Autodesk Inventor part; units mm, degrees
ref_plane "YZ Plane" through (0, 0, 0) normal (1, 0, 0) x (0, 1, 0)
ref_plane "XZ Plane" through (0, 0, 0) normal (0, 1, 0) x (-1, 0, 0)
ref_plane "XY Plane" through (0, 0, 0) normal (0, 0, 1) x (1, 0, 0)
sketch "Esboço1" plane through (0, 0, 0) normal (0, 0, 1) x (1, 0, 0)
  line L0 (555, 651.5) -> (-555, 651.5)
  line L1 (-555, 651.5) -> (-555, -651.5)
  line L2 (-555, -651.5) -> (555, -651.5)
  line L3 (555, -651.5) -> (555, 651.5)
  point P0 (0, 0)
  point P1 (555, 0)
  point P2 (0, 651.5)
  dimension "d11" = 1110
  dimension "d12" = 1303
extrude "Extrusão1" add sketch "Esboço1" against normal blind 1700
sketch "Esboço3" plane through (-555, -651.5, 0) normal (0, -1, 0) x (1, 0, 0)
  line L0 (960, -1400) -> (250, -1400)
  line L1 (250, -1400) -> (250, -840)
  line L2 (250, -840) -> (960, -840)
  line L3 (960, -840) -> (960, -1400)
  line L4 (1110, 0) -> (1110, -1700) construction
  line L5 (0, 0) -> (0, -1700) construction
  line L6 (1110, -1700) -> (0, -1700)
  line L7 (1110, 0) -> (0, 0) construction
  point P0 (555, 0)
  dimension "d2" = 150
  dimension "d3" = 250
  dimension "d4" = 300
  dimension "d10" = 560
  dimension "d17" = 840
extrude "Extrusão2" cut sketch "Esboço3" against normal through all
chamfer "Chanfro2" distance 300 angle 45 1 edges at (555, 0, -1700)
chamfer "Chanfro1" distance 200 angle 45 2 edges at (-305, 0, -1400) (405, 0, -1400)
sketch "Esboço4" plane through (555, -651.5, 0) normal (1, 0, 0) x (0, 0, -1)
  line L0 (0, 1303) -> (0, 0)
  line L1 (660, 952.5) -> (0, 952.5)
  line L2 (0, 952.5) -> (0, 350.5)
  line L3 (0, 350.5) -> (660, 350.5)
  line L4 (660, 350.5) -> (660, 952.5)
  line L5 (0, 1303) -> (1400, 1303)
  line L6 (0, 0) -> (1400, 0)
  point P0 (0, 651.5)
  point P1 (0, 952.5)
  dimension "d19" = 350.5
  dimension "d20" = 350.5
  dimension "d21" = 660
  dimension "d22" = 602
extrude "Extrusão3" cut sketch "Esboço4" against normal blind 300
sketch "Esboço6" plane through (-555, -651.5, 0) normal (-1, 0, 0) x (0, 0, 1)
  line L0 (-660, 349) -> (0, 349)
  line L1 (0, 349) -> (0, 954)
  line L2 (0, 954) -> (-660, 954)
  line L3 (-660, 954) -> (-660, 349)
  line L4 (0, 1303) -> (0, 0)
  line L5 (0, 952.5) -> (-660, 952.5)
  point P0 (0, 651.5)
  point P1 (0, 651.5)
  dimension "d30" = 660
  dimension "d31" = 660
  dimension "d32" = 605
extrude "Extrusão5" cut sketch "Esboço6" against normal blind 300 contours L3 L5 L1 L0
shell "Casca1" thickness 1.5 removed faces 7 at (85, 534.6667, 0) at (168.3333, -217.1667, -840) at (-305, 217.1667, -960) at (-238.3333, -217.1667, -1266.6667) at (-1.6667, -217.1667, -1400) at (405, -217.1667, -1080) at (271.6667, -217.1667, -1333.3333)
sketch "Esboço5" plane through (0, 0, -1700) normal (0, 0, -1) x (-1, 0, 0)
  line L0 (55, 501.5) -> (-555, 501.5)
  line L1 (-555, 501.5) -> (-555, -501.5)
  line L2 (-555, -501.5) -> (55, -501.5)
  line L3 (55, -501.5) -> (55, 501.5)
  line L4 (-255, 651.5) -> (-555, 651.5) construction
  line L5 (-255, -651.5) -> (555, -651.5) construction
  line L6 (-555, 651.5) -> (-555, -651.5) construction
  line L7 (555, -651.5) -> (555, 651.5) construction
  line L8 (555, 651.5) -> (-555, 651.5)
  line L9 (-555, 651.5) -> (-555, -651.5)
  line L10 (-555, -651.5) -> (555, -651.5)
  line L11 (555, -651.5) -> (555, 651.5)
  point P0 (0, 0)
  dimension "d25" = 150
  dimension "d26" = 150
  dimension "d27" = 500
extrude "Extrusão4" cut sketch "Esboço5" against normal blind 800 contours L3 L2 L1 L0
sketch "Esboço7" plane through (255, -651.5, 0) normal (1, 0, 0) x (0, 0, -1)
  line L0 (661.5, 349) -> (0, 349) construction
  line L1 (440, 952.5) -> (435, 952.5)
  line L2 (435, 952.5) -> (435, 349)
  line L3 (435, 349) -> (440, 349)
  line L4 (440, 349) -> (440, 952.5)
  line L5 (0, 952.5) -> (660, 952.5) construction
  line L6 (0, 350.5) -> (0, 952.5) construction
  line L7 (660, 350.5) -> (0, 350.5) construction
  line L8 (660, 952.5) -> (660, 350.5) construction
  line L9 (0, 952.5) -> (660, 952.5)
  line L10 (215, 952.5) -> (210, 952.5)
  line L11 (210, 952.5) -> (210, 350.5)
  line L12 (210, 350.5) -> (215, 350.5)
  line L13 (215, 350.5) -> (215, 952.5)
  point P0 (0, 651.5)
  point P1 (437.5, 952.5)
  dimension "d35" = 5
  dimension "d36" = 220
  dimension "d37" = 220
equation "\"d20\" = d19"
equation "\"d26\" = d25"
equation "\"d36\" = d37"
properties part number "Croqui Célula"
For this review, take the finished solid that the model builds, in its own axes (mm). A direction names the side the tool comes from. Coordinates: 2 decimals unless noted, no trailing zeros. Write each loop counter-clockwise with the first axis right and the second up, starting at its lowest first coordinate (ties: lowest second). Pieces come first, ordered by that corner, then holes.
(1) For pin 1 Ø5 at (y, z) = (48.5, -1328) entering from +X; pin 2 Ø1 at (x, y) = (309, -138.5) entering from +Z; pin 3 Ø1.6 at (y, z) = (-108, -1699) entering from +X, all flat-tipped, find the tip position at first contact; note any pin that passes through.
(2) Add section A-A on y = -157. Give the boundary of the cut face in (x, z), then the cut area to 3 significant figures.
(3) The part is to be moulded in two halves that separate along X. For faces 1 (the face through (401.85, 574.71, -1551.03)), 2 (the face through (-246, 9, -1700)), 3 (the face through (555, -9, -690)), say which applies: +X half, -X half, draft (parallel to the pull), parting line (faces both ways), or undercut.
(4) Add section B-B on z = -1108. Give the boundary of the cut face in (x, y), then the cut area to 3 significant figures.
(5) Add section D-D on z = -326.5. Give the boundary of the cut face in (x, y).
(6) Wall thickness on probe 1 along Y at (x, z) = (-487, -189.5); probe 2 along X at (y, z) = (207, -654); probe 3 along Y at (x, z) = (-104, -93): over which ranges is each line inside the solid? List them lowest first.
(7) Tool access review of faces 4 (the face through (8, 650, -837)), 5 (the face through (406, -302.5, -326)), 6 (the face through (-407, 3, -660)): name each direction out of +Z, -Z, +X, -X, +Y, -Y from which nothing blocks a thin tool from reaching the whole face with its end or side.
(8) Add section C-C on x = -152.5. Give the boundary of the cut face in (y, z).
Answer sheet:
1. pin 1: stops at x = -553.5
1. pin 2: stops at z = -660
1. pin 3: stops at x = -55
2. outline: (-555, -1700) - (-55, -1700) - (-55, -1698.5) - (-553.5, -1698.5) - (-553.5, -661.5) - (-253.5, -661.5) - (-253.5, 0) - (-255, 0) - (-255, -660) - (-555, -660) - close; (253.5, -661.5) - (553.5, -661.5) - (553.5, -900) - (555, -900) - (555, -660) - (255, -660) - (255, 0) - (253.5, 0) - close
2. area: 5,550 mm2
3. face 1: undercut
3. face 2: draft
3. face 3: +X half
4. outline: (-555, -651.5) - (-305, -651.5) - (-305, -650) - (-553.5, -650) - (-553.5, 650) - (-305, 650) - (-305, 651.5) - (-555, 651.5) - close; (405, -651.5) - (555, -651.5) - (555, -501.5) - (553.5, -501.5) - (553.5, -650) - (405, -650) - close; (405, 650) - (553.5, 650) - (553.5, 501.5) - (555, 501.5) - (555, 651.5) - (405, 651.5) - close
4. area: 3,600 mm2
5. outline: (-555, -651.5) - (555, -651.5) - (555, -301) - (255, -301) - (255, 301) - (555, 301) - (555, 651.5) - (-555, 651.5) - (-555, 301) - (-255, 301) - (-255, -302.5) - (-555, -302.5) - close; hole (-553.5, -650) - (553.5, -650) - (553.5, -302.5) - (253.5, -302.5) - (253.5, 302.5) - (553.5, 302.5) - (553.5, 650) - (-553.5, 650) - (-553.5, 302.5) - (-253.5, 302.5) - (-253.5, -304) - (-553.5, -304) - close
6. probe 1: y = -651.5 to -650, -304 to -302.5, 301 to 302.5, 650 to 651.5
6. probe 2: x = -255 to -253.5, 253.5 to 255
6. probe 3: y = -651.5 to -650, 650 to 651.5
7. face 4: +Z
7. face 5: +Z, -Z
7. face 6: +Z, -X
8. outline: (-651.5, -1700) - (651.5, -1700) - (651.5, -1352.5) - (650, -1352.5) - (650, -1698.5) - (-650, -1698.5) - (-650, -1352.5) - (-651.5, -1352.5) - close; (-651.5, -840) - (-650, -840) - (-650, 0) - (-651.5, 0) - close; (650, -840) - (651.5, -840) - (651.5, 0) - (650, 0) - close
